from build123d import *

# Parameters (mm, degrees)
BOSS_EXTRUDE1_DEPTH = 4
CUT_EXTRUDE1_REACH  = 6
SKETCH1_3_R         = 1
SKETCH1_3_R_2       = 1.5
SKETCH1_4_R         = 2.5
CUT_EXTRUDE2_DEPTH  = 2
SKETCH2_R           = 2.5
CUT_EXTRUDE3_DEPTH  = 2


with BuildPart() as part:
    # Sketch1 → Boss-Extrude1 (new body)
    with BuildSketch(Plane(origin=(0, 0, 0), x_dir=(1, 0, 0), z_dir=(0, 1, 0))):
        with BuildLine():
            Line((0, 4), (10, 4))
            ThreePointArc((10, 4), (11.414213562, 3.414213562), (12, 2))
            Line((12, 2), (12, -2))
            ThreePointArc((12, -2), (11.414213562, -3.414213562), (10, -4))
            Line((10, -4), (0, -4))
            Line((0, -4), (-10, -4))
            ThreePointArc((-10, -4), (-11.414213562, -3.414213562), (-12, -2))
            Line((-12, -2), (-12, 2))
            ThreePointArc((-12, 2), (-11.414213562, 3.414213562), (-10, 4))
            Line((-10, 4), (0, 4))
        make_face()
    extrude(amount=BOSS_EXTRUDE1_DEPTH)

    # Sketch1_3 → Cut-Extrude1 (cut, up to next)
    with BuildSketch(Plane(origin=(0, 0, 0), x_dir=(1, 0, 0), z_dir=(0, 1, 0)), mode=Mode.PRIVATE) as cut_extrude1_sk1:
        Circle(SKETCH1_3_R)
    cut_extrude1_tool1 = extrude(cut_extrude1_sk1.sketch, amount=CUT_EXTRUDE1_REACH, mode=Mode.PRIVATE) & part.part
    add(cut_extrude1_tool1.solids().sort_by_distance((0, 0, 0))[0], mode=Mode.SUBTRACT)
    # Sketch1_3 → Cut-Extrude1 (cut, up to next)
    with BuildSketch(Plane(origin=(0, 0, 0), x_dir=(1, 0, 0), z_dir=(0, 1, 0)), mode=Mode.PRIVATE) as cut_extrude1_sk2:
        with Locations((-7, 0)):
            Circle(SKETCH1_3_R_2)
    cut_extrude1_tool2 = extrude(cut_extrude1_sk2.sketch, amount=CUT_EXTRUDE1_REACH, mode=Mode.PRIVATE) & part.part
    add(cut_extrude1_tool2.solids().sort_by_distance((-7, 0, 0))[0], mode=Mode.SUBTRACT)
    # Sketch1_3 → Cut-Extrude1 (cut, up to next)
    with BuildSketch(Plane(origin=(0, 0, 0), x_dir=(1, 0, 0), z_dir=(0, 1, 0)), mode=Mode.PRIVATE) as cut_extrude1_sk3:
        with Locations((7, 0)):
            Circle(SKETCH1_3_R_2)
    cut_extrude1_tool3 = extrude(cut_extrude1_sk3.sketch, amount=CUT_EXTRUDE1_REACH, mode=Mode.PRIVATE) & part.part
    add(cut_extrude1_tool3.solids().sort_by_distance((7, 0, 0))[0], mode=Mode.SUBTRACT)

    # Sketch1_4 → Cut-Extrude2 (cut)
    with BuildSketch(Plane(origin=(0, 0, 0), x_dir=(1, 0, 0), z_dir=(0, 1, 0))):
        Circle(SKETCH1_4_R)
    extrude(amount=CUT_EXTRUDE2_DEPTH, mode=Mode.SUBTRACT)

    # Sketch2 → Cut-Extrude3 (cut)
    with BuildSketch(Plane(origin=(0, 4, 0), x_dir=(1, 0, 0), z_dir=(0, 1, 0))):
        with Locations((-7, 0)):
            Circle(SKETCH2_R)
        with Locations((7, 0)):
            Circle(SKETCH2_R)
    extrude(amount=-CUT_EXTRUDE3_DEPTH, mode=Mode.SUBTRACT)


solid = part.part
Work out the finished part from the listing and answer in its coordinate system (mm). A direction names the side the tool comes from. Give positions to 0.01 mm unless a question says otherwise; leave off trailing zeros. Order: outer loops, then holes, each group sorted by start corner. A loop starts at its lowest first (then second) coordinate and runs counter-clockwise, first axis right, second up. Notation, with made-up numbers: (-10, -7) -> (8, -7) arc R18 ccw to (8, 5) -> close; hole circle Ø2 at (1.25, 51). An arc over 180 degrees is marked (long way). Answer as a JSON object with one key per item and string values. Group by question number.
1. Section C-C on y = 1.65 is taken. Determine the outline of the cut face in (x, z), plus the area to 3 significant figures.
2. Flat-ended cylindrical pins translate along their axes: pin 1 Ø4 at (x, z) = (7, 0) entering from -Y; pin 2 Ø1.8 at (x, z) = (0, 0) entering from -Y; pin 3 Ø1.5 at (x, z) = (-8, 0.5) entering from +Y. Find the tip coordinate at first contact, or state that the pin passes through.
3. Consider line 1 along X through (y, z) = (0.65, 0); line 2 along Z through (x, y) = (7, 2.5); line 3 along Z through (x, y) = (0, 2.5). Determine where each line is inside the solid, lowest interval first. Write a range as [from, to].
4. A tool of negligible diameter and unlimited length cuts with its end or side. For faces 1 (the cylindrical face through (-0.54, 0.99, 2.44)), 2 (the cylindrical face through (5.5, 0.99, -0.07)), 3 (the cylindrical face through (-4.615, 3.014, -0.751)), from which of +Z, -Z, +X, -X, +Y, -Y can it reach the whole face along a straight path? Write none if from no direction.
5. Section B-B on x = -7 is taken. Determine the outline of the cut face in (y, z), plus the area to 3 significant figures.
6. Section D-D on x = 1.5 is taken. Determine the outline of the cut face in (y, z), plus the area to 3 significant figures.
7. Section A-A on z = 0 is taken. Determine the outline of the cut face in (x, y), plus the area to 3 significant figures.
Result sheet:
{
 "1": {"outline": "(-12, -2) arc R2 ccw to (-10, -4) -> (10, -4) arc R2 ccw to (12, -2) -> (12, 2) arc R2 ccw to (10, 4) -> (-10, 4) arc R2 ccw to (-12, 2) -> close; hole circle Ø3 at (-7, 0); hole circle Ø5 at (0, 0); hole circle Ø3 at (7, 0)", "area": "155 mm^2"},
 "2": {"pin 1": "stops at y = 0", "pin 2": "passes through", "pin 3": "stops at y = 2"},
 "3": {"line 1": "x = [-12, -8.5], [-5.5, -2.5], [2.5, 5.5], [8.5, 12]", "line 2": "z = [-4, -2.5], [2.5, 4]", "line 3": "z = [-4, -1], [1, 4]"},
 "4": {"face 1": "-Y", "face 2": "+Y, -Y", "face 3": "+Y"},
 "5": {"outline": "(0, -4) -> (4, -4) -> (4, -2.5) -> (2, -2.5) -> (2, -1.5) -> (0, -1.5) -> close; (0, 1.5) -> (2, 1.5) -> (2, 2.5) -> (4, 2.5) -> (4, 4) -> (0, 4) -> close", "area": "16.0 mm^2"},
 "6": {"outline": "(0, -4) -> (4, -4) -> (4, 4) -> (0, 4) -> (0, 2) -> (2, 2) -> (2, -2) -> (0, -2) -> close", "area": "24.0 mm^2"},
 "7": {"outline": "(-12, 0) -> (-8.5, 0) -> (-8.5, 2) -> (-9.5, 2) -> (-9.5, 4) -> (-12, 4) -> close; (-5.5, 0) -> (-2.5, 0) -> (-2.5, 2) -> (-1, 2) -> (-1, 4) -> (-4.5, 4) -> (-4.5, 2) -> (-5.5, 2) -> close; (1, 2) -> (2.5, 2) -> (2.5, 0) -> (5.5, 0) -> (5.5, 2) -> (4.5, 2) -> (4.5, 4) -> (1, 4) -> close; (8.5, 0) -> (12, 0) -> (12, 4) -> (9.5, 4) -> (9.5, 2) -> (8.5, 2) -> close", "area": "50.0 mm^2"}
}
